Verification items for the finished model (mm, model axes). Face numbers are marked on the shaded views. A direction names the side the tool comes from. Give positions to 0.01 mm unless a question says otherwise; leave off trailing zeros. Order: outer loops, then holes, each group sorted by start corner. A loop starts at its lowest first (then second) coordinate and runs counter-clockwise, first axis right, second up.
from build123d import *

# Parameters (mm, degrees)
F0_R     = 7.5
F0_R_2   = 2.25
F1_DEPTH = 1
F2_R     = 5.5
F2_R_2   = 2.25
F3_DEPTH = 6
F4_R     = 7.5
F4_R_2   = 2.25
F5_DEPTH = 1


with BuildPart() as f1:
    # F0 (on Front) → F1 (new body)
    with BuildSketch(Plane.XZ):
        Circle(F0_R)
        Circle(F0_R_2, mode=Mode.SUBTRACT)
    extrude(amount=-F1_DEPTH)

    # F2 (on face) → F3 (join)
    with BuildSketch(Plane.XZ):
        Circle(F2_R)
        Circle(F2_R_2, mode=Mode.SUBTRACT)
    extrude(amount=F3_DEPTH)

    # F4 (on face) → F5 (join)
    with BuildSketch(Plane.XZ.offset(6)):
        Circle(F4_R)
        Circle(F4_R_2, mode=Mode.SUBTRACT)
    extrude(amount=F5_DEPTH)


solid = f1.part
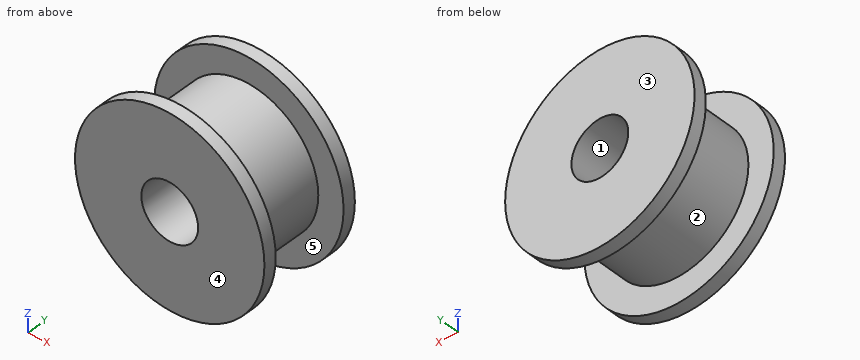
(1) Section check C-C, the plane y = -1. Enter the section's corners in (x, z).
Solved:
outline: circle Ø11 at (0, 0); hole circle Ø4.5 at (0, 0)
(2) Section check D-D, the plane z = 2.75. Enter the section's corners in (x, y).
Solved:
outline: (-6.98, -7) - (6.98, -7) - (6.98, -6) - (4.76, -6) - (4.76, 0) - (6.98, 0) - (6.98, 1) - (-6.98, 1) - (-6.98, 0) - (-4.76, 0) - (-4.76, -6) - (-6.98, -6) - close
(3) Go/stop test with flat-tipped pins: pin 1 (3 mm diameter, centred on x = 1.5, y = -2.5, fed in from +Z); pin 2 (4 mm diameter, centred on x = 0, z = 0, fed in from -Y). Record where each tip stops, or that it passes through.
Solved:
pin 1: stops at z = 5.5
pin 2: passes through
(4) Section check B-B, the plane z = 0. Enter the section's corners in (x, y).
Solved:
outline: (-7.5, -7) - (-2.25, -7) - (-2.25, 1) - (-7.5, 1) - (-7.5, 0) - (-5.5, 0) - (-5.5, -6) - (-7.5, -6) - close; (2.25, -7) - (7.5, -7) - (7.5, -6) - (5.5, -6) - (5.5, 0) - (7.5, 0) - (7.5, 1) - (2.25, 1) - close
(5) Release check for a two-part mould opening along Y. For the marked faces 3, 4 and 5 record: pulls with the +Y half, pulls with the -Y half, needs draft (parallel to the pull), parting line crosses it, or undercut.
Solved:
face 3: pulls with the +Y half
face 4: pulls with the -Y half
face 5: undercut
(6) Section check A-A, the plane x = 0. Enter the section's corners in (y, z), then the cut area to 3 significant figures.
Solved:
outline: (-7, -7.5) - (-6, -7.5) - (-6, -5.5) - (0, -5.5) - (0, -7.5) - (1, -7.5) - (1, -2.25) - (-7, -2.25) - close; (-7, 2.25) - (1, 2.25) - (1, 7.5) - (0, 7.5) - (0, 5.5) - (-6, 5.5) - (-6, 7.5) - (-7, 7.5) - close
area: 60.0 mm2
(7) Set-up check for the marked faces 1 and 2: record each of +Z, -Z, +X, -X, +Y, -Y from which the full face is reachable in a straight line by a thin tool's end or side.
Solved:
face 1: +Y, -Y
face 2: none
(8) Scan lines: line 1 (Y direction, x = -6.75, z = -0.5); line 2 (Z direction, x = 0, y = -2); line 3 (X direction, y = -2.5, z = 1.5). Record each from-to range of solid material in increasing order.
Solved:
line 1: y = -7 to -6, 0 to 1
line 2: z = -5.5 to -2.25, 2.25 to 5.5
line 3: x = -5.29 to -1.68, 1.68 to 5.29
